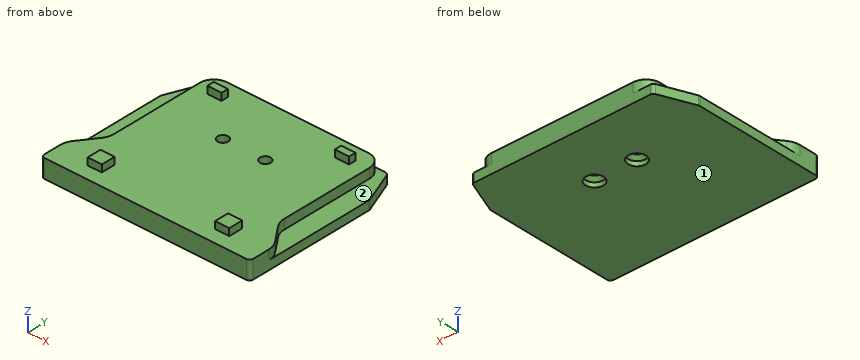
from build123d import *

# Parameters (mm, degrees)
F1_DEPTH      = 2.5
F3_DEPTH      = 2.7
F4_R          = 1
F5_R          = 5
F6_W          = 4
F6_H          = 2
F6_H_2        = 4
F7_DEPTH      = 2
F8_R          = 1.5
F9_DEPTH      = 6
F10_R         = 2.5
F11_DEPTH     = 2.5
F12_S5_R      = 1.5
F12_T6_DEPTH  = 5
F12_S11_R     = 1.5
F12_T12_DEPTH = 5


# Not quite as in the source:
# - a fillet or chamfer that OpenCascade refuses, or shapes differently, is made with other operations: its cross-section is extruded or revolved along the edge and cut away or added


with BuildPart() as f1:
    # F0 (on Top) → F1 (new body)
    with BuildSketch(Plane.XY):
        Polygon((55, 0), (4, 0), (0, -10), (0, -47), (59, -47), (59, -10), align=None)
    extrude(amount=F1_DEPTH)

    # F2 (on face) → F3 (join)
    with BuildSketch(Plane.XY.offset(2.5)):
        with BuildLine():
            Line((0, -39.5), (0, -47))
            Line((0, -47), (59, -47))
            Line((59, -47), (59, -39.5))
            Line((59, -39.5), (53.5, -32))
            Line((53.5, -32), (53.5, -4))
            ThreePointArc((53.5, -4), (52.3284271247, -1.1715728753), (49.5, 0))
            Line((49.5, 0), (9.5, 0))
            ThreePointArc((9.5, 0), (6.6715728753, -1.1715728753), (5.5, -4))
            Line((5.5, -4), (5.5, -32))
            Line((5.5, -32), (0, -39.5))
        make_face()
    extrude(amount=F3_DEPTH)

    # F4
    f4_edges = [f1.edges().sort_by_distance(p)[0] for p in [
        (0, -47, 2.6),
        (59, -47, 2.6),
        (4, 0, 1.25),
        (55, 0, 1.25),
        (59, -10, 1.25),
        (0, -10, 1.25),
    ]]
    fillet(f4_edges, radius=F4_R)

    # F5
    f5_edges = [f1.edges().sort_by_distance(p)[0] for p in [
        (0, -39.5, 3.85),
        (59, -39.5, 3.85),
        (53.5, -32, 3.85),
        (5.5, -32, 3.85),
    ]]
    fillet(f5_edges, radius=F5_R)

    # F6 (on face) → F7 (join)
    with BuildSketch(Plane.XY.offset(5.2)):
        with Locations((11.5, -5)):
            Rectangle(F6_W, F6_H)
        with Locations((11.5, -41)):
            Rectangle(F6_W, F6_H_2)
        with Locations((47.5, -5)):
            Rectangle(F6_W, F6_H)
        with Locations((47.5, -41)):
            Rectangle(F6_W, F6_H_2)
    extrude(amount=F7_DEPTH)

    # F8 (on face) → F9 (cut)
    with BuildSketch(Plane.XY.offset(5.2)):
        with Locations((23.5, -16.5)):
            Circle(F8_R)
        with Locations((35.5, -16.5)):
            Circle(F8_R)
    extrude(amount=-F9_DEPTH, mode=Mode.SUBTRACT)

    # F10 (on face) → F11 (cut)
    with BuildSketch(Plane.XY):
        with Locations((35.5, -16.5)):
            Circle(F10_R)
        with Locations((23.5, -16.5)):
            Circle(F10_R)
    extrude(amount=F11_DEPTH, mode=Mode.SUBTRACT)

    # F12: chamfer of 1.2 on 2 edges, made by hand


with BuildPart() as f12_tool2:
    # F12_s3 → F12_t4 (revolve)
    with BuildSketch(Plane.XZ.offset(16.5)):
        Polygon((38, 1.3), (36.8, 2.5), (38, 2.5), align=None)
    revolve(axis=Axis((35.5, -16.5, 2.5), (0, 0, 1)))

    # F12_s5 → F12_t6 (cut, symmetric)
    with BuildSketch(Plane.XY.offset(1.9)):
        with Locations((35.5, -16.5)):
            Circle(F12_S5_R)
    extrude(amount=F12_T6_DEPTH, both=True, mode=Mode.SUBTRACT)


with BuildPart() as f1_1:
    add(f1.part)

    # F12_t1: union F12_tool2
    add(f12_tool2.part)


with BuildPart() as f12_tool8:
    # F12_s9 → F12_t10 (revolve)
    with BuildSketch(Plane.XZ.offset(16.5)):
        Polygon((26, 1.3), (24.8, 2.5), (26, 2.5), align=None)
    revolve(axis=Axis((23.5, -16.5, 2.5), (0, 0, 1)))

    # F12_s11 → F12_t12 (cut, symmetric)
    with BuildSketch(Plane.XY.offset(1.9)):
        with Locations((23.5, -16.5)):
            Circle(F12_S11_R)
    extrude(amount=F12_T12_DEPTH, both=True, mode=Mode.SUBTRACT)


with BuildPart() as f1_2:
    add(f1_1.part)

    # F12_t7: union F12_tool8
    add(f12_tool8.part)


solid = f1_2.part
Here's how the part is built. I have some questions about the finished solid (model axes, mm). Face numbers are marked on the shaded views. A direction names the side the tool comes from. Round coordinates to 2 decimals unless told otherwise and drop trailing zeros. Loops run counter-clockwise (first coordinate to the right, second up) from the corner with the lowest first, then second, coordinate; pieces in that order, holes last. Notation, with made-up numbers: (77.5, 33) -> (125.5, 33) arc R25 cw to (125.5, 67) -> close; hole circle Ø10 at (-0.75, 28.25). An arc over 180 degrees is marked (long way). Write each question's results on one line, items separated by ' | '.
(1) If I drill on L1, parallel to Y at x = 35.5, z = 3.05; L2, parallel to X at y = -15, z = 1.75; L3, parallel to Y at x = 35.5, z = 0.5, over which ranges is the centre line in solid material (lowest first)?
Worked answers:
L1: -47 to -18, -15 to 0 | L2: 0 to 22.1, 24.9 to 34.1, 36.9 to 59 | L3: -47 to -19, -14 to 0
(2) For the marked faces 1 and 2, which set-ups out of +Z, -Z, +X, -X, +Y, -Y let a thin tool reach every point of the face, with its end or its side?
Worked answers:
face 1: -Z, +X, -X, +Y, -Y | face 2: +Z, +X, +Y
(3) If we section it at C-C, the plane y = -16.5: List the corners of the cut face in (x, z) for me, then the cut area to 3 significant figures.
Worked answers:
outline: (0, 0) -> (21, 0) -> (21, 1.3) -> (22, 2.3) -> (22, 5.2) -> (5.5, 5.2) -> (5.5, 2.5) -> (0, 2.5) -> close; (25, 2.3) -> (26, 1.3) -> (26, 0) -> (33, 0) -> (33, 1.3) -> (34, 2.3) -> (34, 5.2) -> (25, 5.2) -> close; (37, 2.3) -> (38, 1.3) -> (38, 0) -> (59, 0) -> (59, 2.5) -> (53.5, 2.5) -> (53.5, 5.2) -> (37, 5.2) -> close | area: 239 mm2
(4) For P1, Ø0.6, axis at y = -4.5, z = 6, coming from the -X side; P2, Ø8, axis at x = 23.5, y = -16.5, coming from the +Z side; P3, Ø0.6, axis at x = 12.5, z = 6, coming from the -Y side; P4, Ø2.5, axis at x = 35.5, y = -16.5, coming from the +Z side, each with a flat end and sliding along its axis, tell me the tip position at first contact or that it passes through.
Worked answers:
P1: x = 9.5 | P2: z = 5.2 | P3: y = -43 | P4: through
(5) If we section it at A-A, the plane z = 6.25: List the corners of the cut face in (x, y) for me.
Worked answers:
outline: (9.5, -43) -> (13.5, -43) -> (13.5, -39) -> (9.5, -39) -> close; (9.5, -6) -> (13.5, -6) -> (13.5, -4) -> (9.5, -4) -> close; (45.5, -43) -> (49.5, -43) -> (49.5, -39) -> (45.5, -39) -> close; (45.5, -6) -> (49.5, -6) -> (49.5, -4) -> (45.5, -4) -> close
(6) If we section it at D-D, the plane y = -36.5: List the corners of the cut face in (x, z) for me.
Worked answers:
outline: (0, 0) -> (59, 0) -> (59, 2.5) -> (56.8, 2.5) -> (56.8, 5.2) -> (2.2, 5.2) -> (2.2, 2.5) -> (0, 2.5) -> close
(7) If we section it at B-B, the plane x = 35.5: List the corners of the cut face in (y, z) for me, then the cut area to 3 significant figures.
Worked answers:
outline: (-47, 0) -> (-19, 0) -> (-19, 1.3) -> (-18, 2.3) -> (-18, 5.2) -> (-47, 5.2) -> close; (-15, 2.3) -> (-14, 1.3) -> (-14, 0) -> (0, 0) -> (0, 5.2) -> (-15, 5.2) -> close | area: 225 mm2
